```python
from build123d import *

# Parameters (mm, degrees)
F1_DEPTH = 24
F3_DEPTH = 11.001
F4_DEPTH = 25.8


# Not quite as in the source:
# - a feature names something its author has since deleted; it is built from what else it names


with BuildPart() as f1:
    # F0 (on Right) → F1 (new body, symmetric)
    with BuildSketch(Plane.YZ):
        Polygon((-56, 3.0059725977), (-56, 0), (51, 0), (51, 11), (-29.9936849624, 11), align=None)
    extrude(amount=F1_DEPTH, both=True)

    # F2 (on Top) → F3 (cut, through all)
    with BuildSketch(Plane.XY):
        with BuildLine():
            ThreePointArc((-6.8629677407, 24.5349109173), (0, 17.6719431765), (6.8629677407, 24.5349109173))
            Line((6.8629677407, 24.5349109173), (-6.8629677407, 24.5349109173))
        make_face()
        with BuildLine():
            Line((-6.8629677407, 24.5349109173), (6.8629677407, 24.5349109173))
            ThreePointArc((6.8629677407, 24.5349109173), (0, 31.397878658), (-6.8629677407, 24.5349109173))
        make_face()
        with BuildLine():
            Line((6.8629677407, -24.5349109173), (6.8629677407, 24.5349109173))
            ThreePointArc((6.8629677407, 24.5349109173), (0, 17.6719431765), (-6.8629677407, 24.5349109173))
            Line((-6.8629677407, 24.5349109173), (-6.8629677407, -24.5349109173))
            ThreePointArc((-6.8629677407, -24.5349109173), (0, -17.6719431765), (6.8629677407, -24.5349109173))
        make_face()
        with BuildLine():
            ThreePointArc((-6.8629677407, -24.5349109173), (0, -31.397878658), (6.8629677407, -24.5349109173))
            Line((6.8629677407, -24.5349109173), (-6.8629677407, -24.5349109173))
        make_face()
        with BuildLine():
            Line((-6.8629677407, -24.5349109173), (6.8629677407, -24.5349109173))
            ThreePointArc((6.8629677407, -24.5349109173), (0, -17.6719431765), (-6.8629677407, -24.5349109173))
        make_face()
    extrude(amount=F3_DEPTH, mode=Mode.SUBTRACT)

    # F2 (on Top) → F4 (cut)
    with BuildSketch(Plane.XY):
        with BuildLine():
            ThreePointArc((-6.8629677407, 24.5349109173), (0, 17.6719431765), (6.8629677407, 24.5349109173))
            Line((6.8629677407, 24.5349109173), (-6.8629677407, 24.5349109173))
        make_face()
        with BuildLine():
            Line((-6.8629677407, 24.5349109173), (6.8629677407, 24.5349109173))
            ThreePointArc((6.8629677407, 24.5349109173), (0, 31.397878658), (-6.8629677407, 24.5349109173))
        make_face()
        with BuildLine():
            Line((6.8629677407, -24.5349109173), (6.8629677407, 24.5349109173))
            ThreePointArc((6.8629677407, 24.5349109173), (0, 17.6719431765), (-6.8629677407, 24.5349109173))
            Line((-6.8629677407, 24.5349109173), (-6.8629677407, -24.5349109173))
            ThreePointArc((-6.8629677407, -24.5349109173), (0, -17.6719431765), (6.8629677407, -24.5349109173))
        make_face()
        with BuildLine():
            ThreePointArc((-6.8629677407, -24.5349109173), (0, -31.397878658), (6.8629677407, -24.5349109173))
            Line((6.8629677407, -24.5349109173), (-6.8629677407, -24.5349109173))
        make_face()
        with BuildLine():
            Line((-6.8629677407, -24.5349109173), (6.8629677407, -24.5349109173))
            ThreePointArc((6.8629677407, -24.5349109173), (0, -17.6719431765), (-6.8629677407, -24.5349109173))
        make_face()
    extrude(amount=F4_DEPTH, mode=Mode.SUBTRACT)


solid = f1.part
```
The listing builds one solid part. Answer for the finished solid, in the listing's coordinates (mm). A direction names the side the tool comes from. Coordinates: 2 decimals unless noted, no trailing zeros. Write each loop counter-clockwise with the first axis right and the second up, starting at its lowest first coordinate (ties: lowest second). Pieces come first, ordered by that corner, then holes. Notation, with made-up numbers: (77, 21.25) - (119, 21.25) arc R10 ccw to (119, 25.25) - close; hole circle Ø3 at (14.25, -37). An arc over 180 degrees is marked (long way). Return JSON: item names as keys, results as strings. Group by question number.
1. Given pin 1 (1 mm diameter, centred on y = -43, z = 9.5, fed in from -X); pin 2 (10 mm diameter, centred on x = 4, y = -38, fed in from +Z), each flat-ended and moving along its own axis, determine where each tip first touches the part or whether it passes through.
2. A cutting plane is placed at B-B, the plane x = -2. Determine the outline of the cut face in (y, z), plus the area to 3 significant figures.
3. Determine the mould class of faces 1 (the flat face through (11, 11, 11)), 2 (the flat face through (-24, -3, 6)), 3 (the cylindrical face through (-0.151, -31.396, 5.423)), 4 (the cylindrical face through (0.151, 31.396, 5.423)) for opening direction X: released by +X, released by -X, zero draft, split by the parting line, or undercut.
4. Straight lines are drawn through the part: L1, parallel to X at y = 15, z = 10.25; L2, parallel to X at y = 27, z = 7.75; L3, parallel to Y at x = 5, z = 1.5. For each, find the intervals that lie inside material, in ascending order.
5. A cutting plane is placed at A-A, the plane y = -10. Determine the outline of the cut face in (x, z), plus the area to 3 significant figures.
6. A cutting plane is placed at D-D, the plane z = 5. Determine the outline of the cut face in (x, y), plus the area to 3 significant figures.
7. Which of the six approach directions +Z, -Z, +X, -X, +Y, -Y give full straight-line access (tool end or side, diameter ignored) to faces 5 (the flat face through (0, -43, 7)), 6 (the flat face through (6.863, 0, 5))?
8. A cutting plane is placed at C-C, the plane x = 17.5. Determine the outline of the cut face in (y, z), plus the area to 3 significant figures.
Ans:
{
 "1": {"pin 1": "through", "pin 2": "z = 10.08"},
 "2": {"outline": "(-56, 0) - (-31.1, 0) - (-31.1, 10.66) - (-56, 3.01) - close; (31.1, 0) - (51, 0) - (51, 11) - (31.1, 11) - close", "area": "389 mm²"},
 "3": {"face 1": "zero draft", "face 2": "released by -X", "face 3": "undercut", "face 4": "undercut"},
 "4": {"L1": "-24 to -6.86, 6.86 to 24", "L2": "-24 to -6.4, 6.4 to 24", "L3": "-56 to -29.24, 29.24 to 51"},
 "5": {"outline": "(-24, 0) - (-6.86, 0) - (-6.86, 11) - (-24, 11) - close; (6.86, 0) - (24, 0) - (24, 11) - (6.86, 11) - close", "area": "377 mm²"},
 "6": {"outline": "(-24, -49.51) - (24, -49.51) - (24, 51) - (-24, 51) - close; hole (-6.86, -24.53) arc R6.86 ccw to (6.86, -24.53) - (6.86, 24.53) arc R6.86 ccw to (-6.86, 24.53) - close", "area": "4,000 mm²"},
 "7": {"face 5": "+Z, +X, -X, -Y", "face 6": "+Z, -Z"},
 "8": {"outline": "(-56, 0) - (51, 0) - (51, 11) - (-29.99, 11) - (-56, 3.01) - close", "area": "1,070 mm²"}
}
